```python
from build123d import *

# Parameters (mm, degrees)
SKETCH1_R           = 19.05
SKETCH1_R_2         = 12.7
BOSS_EXTRUDE1_DEPTH = 8.46582
BOSS_EXTRUDE2_DEPTH = 8.46582
CIRPATTERN1_COUNT   = 18
FILLET2_R           = 7.62


with BuildPart() as part:
    # Sketch1 → Boss-Extrude1 (new body)
    with BuildSketch(Plane(origin=(0, 0, 0), x_dir=(1, 0, 0), z_dir=(0, 1, 0))):
        with Locations(Location((0, 0, 0), (0, 0, 270))):
            Circle(SKETCH1_R)
        with Locations(Location((0, 0, 0), (0, 0, 270))):
            Circle(SKETCH1_R_2, mode=Mode.SUBTRACT)
    extrude(amount=BOSS_EXTRUDE1_DEPTH)

    # Sketch2 → Boss-Extrude2 (add)
    with BuildSketch(Plane(origin=(0, 0, 0), x_dir=(1, 0, 0), z_dir=(0, 1, 0))):
        with BuildLine():
            Line((-1.778, 18.966845178), (-1.778, 22.141845178))
            Line((-1.778, 22.141845178), (-0.3175, 24.046845178))
            Line((-0.3175, 24.046845178), (0.3175, 24.046845178))
            Line((0.3175, 24.046845178), (1.778, 22.141845178))
            Line((1.778, 22.141845178), (1.778, 18.966845178))
            ThreePointArc((1.778, 18.966845178), (0, 19.05), (-1.778, 18.966845178))
        make_face()
    boss_extrude2 = extrude(amount=BOSS_EXTRUDE2_DEPTH)

    # CirPattern1: Boss-Extrude2 ×18 about axis
    cirpattern1_axis = Axis((0, 0, 0), (0, 1, 0))
    for i in range(1, CIRPATTERN1_COUNT):
        add(boss_extrude2.rotate(cirpattern1_axis, i * 360 / CIRPATTERN1_COUNT))

    # Fillet2
    # the kernel refuses this fillet: 7.62 mm, written as the material it takes off along each edge
    with BuildSketch(Plane(origin=(1.778, -6.452712813, -22.141845178), x_dir=(0, 0, 1), z_dir=(0, 1, 0)), Plane(origin=(20.064400411, -6.452712813, -9.531129421), x_dir=(-0.8660254037844388, 0, 0.49999999999999956), z_dir=(0, 1, 0)), Plane(origin=(22.114207257, -6.452712813, -2.09390288), x_dir=(-0.9848077530122081, 0, 0.17364817766693005), z_dir=(0, 1, 0)), Plane(origin=(21.496714337, -6.452712813, 5.59587925), x_dir=(-0.9848077530122081, 0, -0.17364817766692997), z_dir=(0, 1, 0)), Plane(origin=(18.286400411, -6.452712813, 12.610715757), x_dir=(-0.8660254037844383, 0, -0.5000000000000006), z_dir=(0, 1, 0)), Plane(origin=(12.870476716, -6.452712813, 18.104513829), x_dir=(-0.6427876096865391, 0, -0.7660444431189781), z_dir=(0, 1, 0)), Plane(origin=(5.902183581, -6.452712813, 21.414640339), x_dir=(-0.34202014332566927, 0, -0.9396926207859082), z_dir=(0, 1, 0)), Plane(origin=(-1.778, -6.452712813, 22.141845178), x_dir=(0, 0, -1), z_dir=(0, 1, 0)), Plane(origin=(-9.243730541, -6.452712813, 20.198416709), x_dir=(0.34202014332566927, 0, -0.9396926207859082), z_dir=(0, 1, 0)), Plane(origin=(-15.594530756, -6.452712813, 15.818761089), x_dir=(0.6427876096865394, 0, -0.7660444431189781), z_dir=(0, 1, 0)), Plane(origin=(-20.064400411, -6.452712813, 9.531129421), x_dir=(0.8660254037844388, 0, -0.49999999999999956), z_dir=(0, 1, 0)), Plane(origin=(-22.114207257, -6.452712813, 2.09390288), x_dir=(0.984807753012208, 0, -0.17364817766693053), z_dir=(0, 1, 0)), Plane(origin=(-21.496714337, -6.452712813, -5.59587925), x_dir=(0.9848077530122081, 0, 0.17364817766693055), z_dir=(0, 1, 0)), Plane(origin=(15.594530756, -6.452712813, -15.818761089), x_dir=(-0.6427876096865398, 0, 0.7660444431189776), z_dir=(0, 1, 0)), Plane(origin=(-18.286400411, -6.452712813, -12.610715757), x_dir=(0.8660254037844386, 0, 0.5000000000000001), z_dir=(0, 1, 0)), Plane(origin=(-12.870476716, -6.452712813, -18.104513829), x_dir=(0.642787609686539, 0, 0.7660444431189781), z_dir=(0, 1, 0)), Plane(origin=(9.243730541, -6.452712813, -20.198416709), x_dir=(-0.3420201433256689, 0, 0.9396926207859084), z_dir=(0, 1, 0)), Plane(origin=(-5.902183581, -6.452712813, -21.414640339), x_dir=(0.3420201433256684, 0, 0.9396926207859084), z_dir=(0, 1, 0))) as fillet2_piece_1:
        with BuildLine():
            CenterArc((2.581085125, -7.62), FILLET2_R, 90, 36.06658826)
            Line((-1.905, -1.4605), (-1.994721703, -1.33731))
            ThreePointArc((-1.994721703, -1.33731), (-1.045224967, -0.609304391), (-0.092724967, 0.120945609))
            Line((-0.092724967, 0.120945609), (0, 0.1524))
            Line((0, 0.1524), (2.581085125, 0.1524))
            Line((2.581085125, 0.1524), (2.581085125, 0))
        make_face()
    extrude(amount=21.371245626, mode=Mode.SUBTRACT)
    with BuildSketch(Plane(origin=(-1.778, -6.452712813, -22.141845178), x_dir=(0.6084315436571524, 0, -0.7936063612919032), z_dir=(0, 1, 0)), Plane(origin=(22.114207257, -6.452712813, 2.09390288), x_dir=(0.6758966686489332, 0, 0.7369963997939708), z_dir=(0, 1, 0)), Plane(origin=(21.496714337, -6.452712813, -5.59587925), x_dir=(0.8872027262312159, 0, 0.4613798029475262), z_dir=(0, 1, 0)), Plane(origin=(20.064400411, -6.452712813, 9.531129421), x_dir=(0.38306749765514664, 0, 0.9237203539168248), z_dir=(0, 1, 0)), Plane(origin=(15.594530756, -6.452712813, 15.818761089), x_dir=(0.04403473296999355, 0, 0.9990300006968066), z_dir=(0, 1, 0)), Plane(origin=(9.243730541, -6.452712813, 20.198416709), x_dir=(-0.30030927039478544, 0, 0.9538418852802342), z_dir=(0, 1, 0)), Plane(origin=(1.778, -6.452712813, 22.141845178), x_dir=(-0.6084315436571494, 0, 0.7936063612919054), z_dir=(0, 1, 0)), Plane(origin=(-5.902183581, -6.452712813, 21.414640339), x_dir=(-0.8431679932612217, 0, 0.5376501977492841), z_dir=(0, 1, 0)), Plane(origin=(-12.870476716, -6.452712813, 18.104513829), x_dir=(-0.9762059390437181, 0, 0.21684548548626165), z_dir=(0, 1, 0)), Plane(origin=(-18.286400411, -6.452712813, 12.610715757), x_dir=(-0.9914990413122959, 0, -0.1301139926249219), z_dir=(0, 1, 0)), Plane(origin=(-21.496714337, -6.452712813, 5.59587925), x_dir=(-0.8872027262312162, 0, -0.4613798029475256), z_dir=(0, 1, 0)), Plane(origin=(-22.114207257, -6.452712813, -2.09390288), x_dir=(-0.675896668648932, 0, -0.7369963997939716), z_dir=(0, 1, 0)), Plane(origin=(-20.064400411, -6.452712813, -9.531129421), x_dir=(-0.3830674976551464, 0, -0.923720353916825), z_dir=(0, 1, 0)), Plane(origin=(-15.594530756, -6.452712813, -15.818761089), x_dir=(-0.04403473296998761, 0, -0.9990300006968068), z_dir=(0, 1, 0)), Plane(origin=(12.870476716, -6.452712813, -18.104513829), x_dir=(0.9762059390437176, 0, -0.21684548548626464), z_dir=(0, 1, 0)), Plane(origin=(18.286400411, -6.452712813, -12.610715757), x_dir=(0.9914990413122965, 0, 0.13011399262491774), z_dir=(0, 1, 0))) as fillet2_piece_2:
        with BuildLine():
            CenterArc((2.587882788, -7.61769408), FILLET2_R, 91.409591302, 36.06658826)
            Line((-2.048365574, -1.570413607), (-2.141090542, -1.449467998))
            Line((-2.141090542, -1.449467998), (-0.092724967, 0.120945609))
            Line((-0.092724967, 0.120945609), (0, 0.1524))
            ThreePointArc((0, 0.1524), (1.200217194, 0.1524), (2.39668542, 0.152353882))
            Line((2.39668542, 0.152353882), (2.400434388, 0))
        make_face()
    extrude(amount=21.371245626, mode=Mode.SUBTRACT)
    with BuildSketch(Plane(origin=(-9.243730541, -6.452712813, -20.198416709), x_dir=(0.34202014332566855, 0, 0.9396926207859084), z_dir=(0, 1, 0)), Plane(origin=(5.902183581, -6.452712813, -21.414640339), x_dir=(-0.34202014332566877, 0, 0.9396926207859084), z_dir=(0, 1, 0))) as fillet2_piece_3:
        with BuildLine():
            CenterArc((2.581085125, 7.62), FILLET2_R, 233.93341174, 36.06658826)
            Line((-1.905, 1.4605), (-1.994721703, 1.33731))
            ThreePointArc((-1.994721703, 1.33731), (-1.045224967, 0.609304391), (-0.092724967, -0.120945609))
            Line((-0.092724967, -0.120945609), (0, -0.1524))
            Line((0, -0.1524), (2.581085125, -0.1524))
            Line((2.581085125, -0.1524), (2.581085125, 0))
        make_face()
    extrude(amount=21.371245626, mode=Mode.SUBTRACT)


solid = part.part
```
Here's how the part is built. I have some questions about the finished solid (model axes, mm). A direction names the side the tool comes from. Give positions to 0.01 mm unless a question says otherwise; leave off trailing zeros. Order: outer loops, then holes, each group sorted by start corner. A loop starts at its lowest first (then second) coordinate and runs counter-clockwise, first axis right, second up. Notation, with made-up numbers: (57, -21) -> (81, -21) arc R19 cw to (81, 1) -> close; hole circle Ø5 at (28.25, 74.5). An arc over 180 degrees is marked (long way). Use CSV: the item, a comma, the result in double quotes. Start each with the question number.
Item 1: Suppose I cut it at B-B (x = -7). List the corners of the cut face in (y, z) for me.
Item 2: I'm going to push flat-ended pins straight in: P1, Ø2, axis at x = 6, y = 4, coming from the +Z side; P2, Ø5, axis at x = -7, y = 1, coming from the -Z side; P3, Ø5, axis at x = 15, y = 2, coming from the +Z side. Where does each tip first touch, or does it pass through?
Item 3: On a 3-axis mill with a long thin cutter (end or side, diameter ignored), from which of +Z, -Z, +X, -X, +Y, -Y can I reach the whole of each face in a straight line? I mean faces 4 (the cylindrical face through (21.8, 4.17, -2.41)), 5 (the cylindrical face through (-21.8, 4.17, 2.41)), 6 (the cylindrical face through (-21.31, 4.174, -5.193)). Say none if no direction works.
Item 4: If I drill on probe 1 along X at (y, z) = (4.25, -21); probe 2 along X at (y, z) = (3.75, -17); probe 3 along X at (y, z) = (4, -8.5), over which ranges is the centre line in solid material (lowest first)? Write a range as [from, to].
Item 5: Thinking about a two-plate mould opening in Z: for faces 1 (the cylindrical face through (-18.25, 4.17, -12.17)), 2 (the cylindrical face through (-14.607, 4.174, 12.229)), 3 (the cylindrical face through (1.393, 4.174, 21.952)), which applies, pulls with the +Z half, pulls with the -Z half, needs draft (parallel to the pull), parting line crosses it, or undercut?
Item 6: Suppose I cut it at A-A (z = 0). List the corners of the cut face in (x, y) for me.
Answer block:
1,outline,"(0, -21.97) -> (8.47, -21.97) -> (8.47, -10.6) -> (0, -10.6) -> close; (0, 10.6) -> (8.47, 10.6) -> (8.47, 21.97) -> (0, 21.97) -> close"
2,P1,"stops at z = 21.97"
2,P2,"stops at z = -22.71"
2,P3,"stops at z = 18.63"
3,face 4,"+X, +Y, -Y"
3,face 5,"-X, +Y, -Y"
3,face 6,"+Y, -Y"
4,probe 1,"x = [-8.8, -6.12], [-1.64, 1.64], [6.12, 8.8]"
4,probe 2,"x = [-15.52, -12.07], [-8.6, 8.6], [12.07, 15.52]"
4,probe 3,"x = [-18.25, -9.44], [9.44, 18.25]"
5,face 1,"pulls with the -Z half"
5,face 2,"undercut"
5,face 3,"pulls with the +Z half"
6,outline,"(-19.05, 0) -> (-12.7, 0) -> (-12.7, 8.47) -> (-19.05, 8.47) -> close; (12.7, 0) -> (19.05, 0) -> (19.05, 8.47) -> (12.7, 8.47) -> close"
